Could you check a few things on this drawing? It's one solid part, dimensions in mm from its lowest x, y, z. A direction names the side the tool comes from. Round coordinates to 2 decimals unless told otherwise and drop trailing zeros. Order: outer loops, then holes, each group sorted by start corner. A loop starts at its lowest first (then second) coordinate and runs counter-clockwise, first axis right, second up.
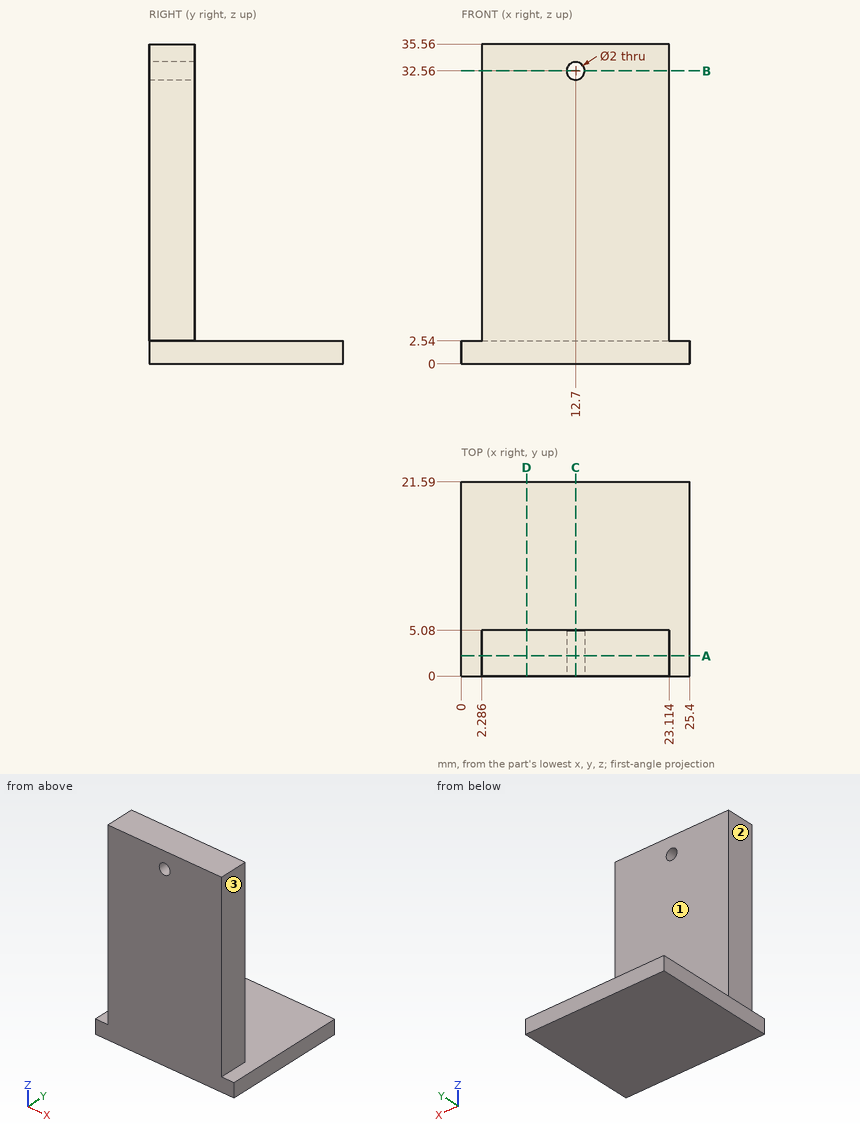
1) If we section it at B-B (z = 32.56): Write out the boundary of the cut face in (x, y).
2) For the marked faces 1, 2 and 3, which set-ups out of +Z, -Z, +X, -X, +Y, -Y let a thin tool reach every point of the face, with its end or its side?
3) I need wall thicknesses on line 1 (X direction, y = 3.05, z = 32.56); line 2 (X direction, y = 3, z = 12.5); line 3 (Z direction, x = 14.5, y = 11.75). Which ranges of each line are inside material? Lowest first, please.
4) I'm going to push flat-ended pins straight in: pin 1 (12 mm diameter, centred on y = 5.5, z = 21.5, fed in from +X); pin 2 (4 mm diameter, centred on y = 2.5, z = 24.5, fed in from -X); pin 3 (1 mm diameter, centred on x = 10.5, z = 29.5, fed in from +Y). Where does each tip first touch, or does it pass through?
5) If we section it at D-D (x = 7.25): Write out the boundary of the cut face in (y, z).
6) If we section it at A-A (y = 2.25): Write out the boundary of the cut face in (x, z), plus the area to 3 significant figures.
7) If we section it at C-C (x = 12.7): Write out the boundary of the cut face in (y, z), plus the area to 3 significant figures.
Solutions:
1. outline: (2.29, 0) - (11.7, 0) - (11.7, 5.08) - (2.29, 5.08) - close; (13.7, 0) - (23.11, 0) - (23.11, 5.08) - (13.7, 5.08) - close
2. face 1: +Z, +X, -X, +Y
2. face 2: +Z, -X, +Y, -Y
2. face 3: +Z, +X, +Y, -Y
3. line 1: x = 2.29 to 11.7, 13.7 to 23.11
3. line 2: x = 2.29 to 23.11
3. line 3: z = 0 to 2.54
4. pin 1: stops at x = 23.11
4. pin 2: stops at x = 2.29
4. pin 3: stops at y = 5.08
5. outline: (0, 0) - (21.59, 0) - (21.59, 2.54) - (5.08, 2.54) - (5.08, 35.56) - (0, 35.56) - close
6. outline: (0, 0) - (25.4, 0) - (25.4, 2.54) - (23.11, 2.54) - (23.11, 35.56) - (2.29, 35.56) - (2.29, 2.54) - (0, 2.54) - close; hole circle Ø2 at (12.7, 32.56)
6. area: 749 mm2
7. outline: (0, 0) - (21.59, 0) - (21.59, 2.54) - (5.08, 2.54) - (5.08, 31.56) - (0, 31.56) - close; (0, 33.56) - (5.08, 33.56) - (5.08, 35.56) - (0, 35.56) - close
7. area: 212 mm2
